Model file for the job. Use its own axes, mm. A direction names the side the tool comes from. Coordinates: 2 decimals unless noted, no trailing zeros. Write each loop counter-clockwise with the first axis right and the second up, starting at its lowest first coordinate (ties: lowest second). Pieces come first, ordered by that corner, then holes. Notation, with made-up numbers: M -32.75,43.25 L 19.25,43.25 A37 ccw 19.25,82.25 Z; hole C 20.5,18 d4. An arc over 180 degrees is marked long. One line per question, with ' | ' between items. Start each with the question number.
(1) Two-plate mould, pull along Y, no slides. Class faces 1 (the face through (132.146, 5.676, -2.465)), 2 (the face through (3.564, 7.535, -3.759)), 3 (the face through (4, 8, -15)): +Y half, -Y half, draft (parallel to the pull), parting line (faces both ways), or undercut.
(2) Tool access for faces 4 (the face through (125, 5, -5)), 5 (the face through (13.4, 9.01, -1.64)), 6 (the face through (25.148, 2.465, -12.751)): list every direction of +Z, -Z, +X, -X, +Y, -Y with a clear straight run to the whole face (end or side of a thin tool).
(3) Flat gauge pins, fed straight in: pin 1 Ø4 at (x, z) = (12.5, -4.5) entering from +Y; pin 2 Ø3.5 at (x, y) = (110, 5) entering from +Z; pin 3 Ø4 at (y, z) = (7.5, -14.5) entering from +X; pin 4 Ø5 at (x, z) = (12.5, -4.5) entering from -Y. Where does each tip first touch, or does it go through?
(4) Wall check: probe 1 along Y at (x, z) = (110, -23.2); probe 2 along Z at (x, y) = (102, 7.25); probe 3 along X at (y, z) = (8.5, -16.75). Give the ranges that are in metal, low to high.
(5) Cut at B-B (z = -16.5). Write the cut outline in (x, y).
(6) Cut at A-A (x = 114.5). Write the cut outline in (y, z), plus the area to 3 significant figures.
from build123d import *

# Parameters (mm, degrees)
SKETCH1_W           = 250
SKETCH1_H           = 25
BOSS_EXTRUDE1_DEPTH = 10
CUT_EXTRUDE1_REACH  = 253.446
SKETCH2_R           = 2.65
FILLET1_R           = 12.5
SKETCH3_R           = 2.25
CUT_EXTRUDE2_DEPTH  = 252.445819214
CUT_EXTRUDE5_REACH  = 253.446
SKETCH5_W           = 7.3
SKETCH5_H           = 4
SKETCH6_R           = 12.65
CUT_EXTRUDE6_DEPTH  = 5
CUT_EXTRUDE7_REACH  = 253.297
SKETCH7_R           = 1.65
SKETCH9_R           = 3
CUT_EXTRUDE9_DEPTH  = 2
CUT_EXTRUDE10_DEPTH = 252.445819214
SKETCH11_R          = 2.25
CUT_EXTRUDE11_DEPTH = 158.321327226


with BuildPart() as part:
    # Sketch1 → Boss-Extrude1 (new body)
    with BuildSketch(Plane(origin=(0, 0, 0), x_dir=(1, 0, 0), z_dir=(0, 1, 0))):
        with Locations((125, 12.5)):
            Rectangle(SKETCH1_W, SKETCH1_H)
    extrude(amount=BOSS_EXTRUDE1_DEPTH)

    # Sketch2 → Cut-Extrude1 (cut, up to next)
    with BuildSketch(Plane(origin=(0, 10, 0), x_dir=(1, 0, 0), z_dir=(0, 1, 0)), mode=Mode.PRIVATE) as cut_extrude1_sk1:
        with Locations(Location((12.5, 12.5, 0), (0, 0, 270))):
            Circle(SKETCH2_R)
    cut_extrude1_tool1 = extrude(cut_extrude1_sk1.sketch, amount=-CUT_EXTRUDE1_REACH, mode=Mode.PRIVATE) & part.part
    add(cut_extrude1_tool1.solids().sort_by_distance((12.5, 10, -12.5))[0], mode=Mode.SUBTRACT)

    # Fillet1
    fillet1_edges = [part.edges().sort_by_distance(p)[0] for p in [
        (0, 5, 0),
        (0, 5, -25),
    ]]
    fillet(fillet1_edges, radius=FILLET1_R - 0.0001)  # a hair under: the kernel refuses the full size

    # Sketch3 → Cut-Extrude2 (cut, through all)
    with BuildSketch(Plane(origin=(0, 0, -25), x_dir=(-1, 0, 0), z_dir=(0, 0, -1))):
        with Locations((-244.5, 5)):
            Circle(SKETCH3_R)
        with Locations((-230.5, 5)):
            Circle(SKETCH3_R)
    extrude(amount=-CUT_EXTRUDE2_DEPTH, mode=Mode.SUBTRACT)

    # Sketch5 → Cut-Extrude5 (cut, up to next)
    with BuildSketch(Plane(origin=(0, 10, 0), x_dir=(1, 0, 0), z_dir=(0, 1, 0)), mode=Mode.PRIVATE) as cut_extrude5_sk1:
        with Locations((244.5, 19)):
            Rectangle(SKETCH5_W, SKETCH5_H)
    cut_extrude5_tool1 = extrude(cut_extrude5_sk1.sketch, amount=-CUT_EXTRUDE5_REACH, mode=Mode.PRIVATE) & part.part
    # Sketch5 → Cut-Extrude5 (cut, up to next)
    with BuildSketch(Plane(origin=(0, 10, 0), x_dir=(1, 0, 0), z_dir=(0, 1, 0)), mode=Mode.PRIVATE) as cut_extrude5_sk2:
        with Locations((244.5, 6)):
            Rectangle(SKETCH5_W, SKETCH5_H)
    cut_extrude5_tool2 = extrude(cut_extrude5_sk2.sketch, amount=-CUT_EXTRUDE5_REACH, mode=Mode.PRIVATE) & part.part
    # Sketch5 → Cut-Extrude5 (cut, up to next)
    with BuildSketch(Plane(origin=(0, 10, 0), x_dir=(1, 0, 0), z_dir=(0, 1, 0)), mode=Mode.PRIVATE) as cut_extrude5_sk3:
        with Locations((230.5, 19)):
            Rectangle(SKETCH5_W, SKETCH5_H)
    cut_extrude5_tool3 = extrude(cut_extrude5_sk3.sketch, amount=-CUT_EXTRUDE5_REACH, mode=Mode.PRIVATE) & part.part
    # Sketch5 → Cut-Extrude5 (cut, up to next)
    with BuildSketch(Plane(origin=(0, 10, 0), x_dir=(1, 0, 0), z_dir=(0, 1, 0)), mode=Mode.PRIVATE) as cut_extrude5_sk4:
        with Locations((230.5, 6)):
            Rectangle(SKETCH5_W, SKETCH5_H)
    cut_extrude5_tool4 = extrude(cut_extrude5_sk4.sketch, amount=-CUT_EXTRUDE5_REACH, mode=Mode.PRIVATE) & part.part
    add(cut_extrude5_tool1.solids().sort_by_distance((244.5, 10, -19))[0], mode=Mode.SUBTRACT)
    add(cut_extrude5_tool2.solids().sort_by_distance((244.5, 10, -6))[0], mode=Mode.SUBTRACT)
    add(cut_extrude5_tool3.solids().sort_by_distance((230.5, 10, -19))[0], mode=Mode.SUBTRACT)
    add(cut_extrude5_tool4.solids().sort_by_distance((230.5, 10, -6))[0], mode=Mode.SUBTRACT)

    # Sketch6 → Cut-Extrude6 (cut)
    with BuildSketch(Plane.XZ):
        with Locations((12.5, -12.5)):
            Circle(SKETCH6_R)
    extrude(amount=-CUT_EXTRUDE6_DEPTH, mode=Mode.SUBTRACT)

    # Sketch7 → Cut-Extrude7 (cut, up to next)
    with BuildSketch(Plane.XZ.offset(-5), mode=Mode.PRIVATE) as cut_extrude7_sk1:
        with Locations(Location((12.5, -4.5, 0), (0, 0, 270))):
            Circle(SKETCH7_R)
    cut_extrude7_tool1 = extrude(cut_extrude7_sk1.sketch, amount=-CUT_EXTRUDE7_REACH, mode=Mode.PRIVATE) & part.part
    # Sketch7 → Cut-Extrude7 (cut, up to next)
    with BuildSketch(Plane.XZ.offset(-5), mode=Mode.PRIVATE) as cut_extrude7_sk2:
        with Locations(Location((19.42820323, -16.5, 0), (0, 0, 270))):
            Circle(SKETCH7_R)
    cut_extrude7_tool2 = extrude(cut_extrude7_sk2.sketch, amount=-CUT_EXTRUDE7_REACH, mode=Mode.PRIVATE) & part.part
    # Sketch7 → Cut-Extrude7 (cut, up to next)
    with BuildSketch(Plane.XZ.offset(-5), mode=Mode.PRIVATE) as cut_extrude7_sk3:
        with Locations(Location((5.57179677, -16.5, 0), (0, 0, 270))):
            Circle(SKETCH7_R)
    cut_extrude7_tool3 = extrude(cut_extrude7_sk3.sketch, amount=-CUT_EXTRUDE7_REACH, mode=Mode.PRIVATE) & part.part
    add(cut_extrude7_tool1.solids().sort_by_distance((12.5, 5, -4.5))[0], mode=Mode.SUBTRACT)
    add(cut_extrude7_tool2.solids().sort_by_distance((19.428203, 5, -16.5))[0], mode=Mode.SUBTRACT)
    add(cut_extrude7_tool3.solids().sort_by_distance((5.571797, 5, -16.5))[0], mode=Mode.SUBTRACT)

    # Sketch9 → Cut-Extrude9 (cut)
    with BuildSketch(Plane(origin=(0, 10, 0), x_dir=(1, 0, 0), z_dir=(0, 1, 0))):
        with Locations(Location((5.57179677, 16.5, 0), (0, 0, 270))):
            Circle(SKETCH9_R)
        with Locations(Location((12.5, 4.5, 0), (0, 0, 270))):
            Circle(SKETCH9_R)
        with Locations(Location((19.42820323, 16.5, 0), (0, 0, 270))):
            Circle(SKETCH9_R)
    extrude(amount=-CUT_EXTRUDE9_DEPTH, mode=Mode.SUBTRACT)

    # Sketch10 → Cut-Extrude10 (cut, through all)
    with BuildSketch(Plane(origin=(0, 10, 0), x_dir=(1, 0, 0), z_dir=(0, 1, 0))):
        Polygon((95, 5), (155, 5), (155, 0), (250, 0), (250, 25), (155, 25), (155, 20), (95, 20), align=None)
    extrude(amount=-CUT_EXTRUDE10_DEPTH, mode=Mode.SUBTRACT)

    # Sketch11 → Cut-Extrude11 (cut, through all)
    with BuildSketch(Plane.XY):
        with Locations((150, 5)):
            Circle(SKETCH11_R)
        with Locations((140, 5)):
            Circle(SKETCH11_R)
        with Locations((130, 5)):
            Circle(SKETCH11_R)
        with Locations((120, 5)):
            Circle(SKETCH11_R)
        with Locations((110, 5)):
            Circle(SKETCH11_R)
    extrude(amount=-CUT_EXTRUDE11_DEPTH, mode=Mode.SUBTRACT)


solid = part.part
Filled in:
1) face 1: undercut | face 2: draft | face 3: +Y half
2) face 4: +X, +Y, -Y | face 5: +Y | face 6: -X, -Y
3) pin 1: y = 8 | pin 2: through | pin 3: x = 95 | pin 4: y = 5
4) probe 1: 0 to 2.75, 7.25 to 10 | probe 2: -25 to -20, -5 to 0 | probe 3: 0.74 to 2.58, 8.56 to 16.44, 22.42 to 95
5) outline: M 0.66,5 L 3.92,5 L 3.92,8 L 2.57,8 L 2.57,10 L 0.66,10 Z; M 7.22,5 L 17.78,5 L 17.78,8 L 16.43,8 L 16.43,10 L 8.57,10 L 8.57,8 L 7.22,8 Z; M 21.08,5 L 24.5,5 L 24.5,0 L 95,0 L 95,10 L 22.43,10 L 22.43,8 L 21.08,8 Z
6) outline: M 0,-25 L 10,-25 L 10,-20 L 0,-20 Z; M 0,-5 L 10,-5 L 10,0 L 0,0 Z | area: 100 mm²
